from build123d import *

# Parameters (mm, degrees)
SKETCH_1_W          = 28
SKETCH_1_H          = 14
EXTRUDE_1_DEPTH     = 14
SKETCH_2_W          = 10
SKETCH_2_H          = 12
CUT_EXTRUDE_1_DEPTH = 25.3
SKETCH_3_R          = 2
CUT_EXTRUDE_2_DEPTH = 25.5
FILLET_4_R          = 2
SKETCH_4_W          = 9.3
SKETCH_4_H          = 14
EXTRUDE_2_DEPTH     = 5
SKETCH_5_W          = 5
SKETCH_5_H          = 14
EXTRUDE_3_DEPTH     = 5
SKETCH_6_R          = 1.48
CUT_EXTRUDE_3_DEPTH = 20


with BuildPart() as part:
    # 草图1 → 凸台-拉伸1 (new body)
    with BuildSketch(Plane(origin=(0, 0, 0), x_dir=(1, 0, 0), z_dir=(0, 1, 0))):
        Rectangle(SKETCH_1_W, SKETCH_1_H)
    extrude(amount=EXTRUDE_1_DEPTH)

    # 草图2 → 切除-拉伸1 (cut)
    with BuildSketch(Plane.ZY.offset(14)):
        with Locations((0, 7)):
            Rectangle(SKETCH_2_W, SKETCH_2_H)
    extrude(amount=-CUT_EXTRUDE_1_DEPTH, mode=Mode.SUBTRACT)

    # 草图3 → 切除-拉伸2 (cut)
    with BuildSketch(Plane(origin=(14, 0, 0), x_dir=(0, 0, -1), z_dir=(1, 0, 0))):
        with Locations((0, 10.5)):
            Circle(SKETCH_3_R)
        with Locations((0, 3.5)):
            Circle(SKETCH_3_R)
    extrude(amount=-CUT_EXTRUDE_2_DEPTH, mode=Mode.SUBTRACT)

    # 圆角4
    fillet_4_edges = [part.edges().sort_by_distance(p)[0] for p in [
        (14, 7, 7),
        (14, 7, -7),
    ]]
    fillet(fillet_4_edges, radius=FILLET_4_R)

    # 草图4 → 凸台-拉伸2 (add)
    with BuildSketch(Plane.XY.offset(7)):
        with Locations((2.35, 7)):
            Rectangle(SKETCH_4_W, SKETCH_4_H)
    extrude(amount=EXTRUDE_2_DEPTH)

    # 草图5 → 凸台-拉伸3 (add)
    with BuildSketch(Plane(origin=(0, 0, -7), x_dir=(-1, 0, 0), z_dir=(0, 0, -1))):
        with Locations((1.8, 7)):
            Rectangle(SKETCH_5_W, SKETCH_5_H)
    extrude(amount=EXTRUDE_3_DEPTH)

    # 草图6 → 切除-拉伸3 (cut)
    with BuildSketch(Plane(origin=(0, 14, 0), x_dir=(1, 0, 0), z_dir=(0, 1, 0))):
        with Locations(Location((2.7, -8.5, 0), (0, 0, 270))):
            Circle(SKETCH_6_R)
        with Locations(Location((-1.8, 8.5, 0), (0, 0, 270))):
            Circle(SKETCH_6_R)
    extrude(amount=-CUT_EXTRUDE_3_DEPTH, mode=Mode.SUBTRACT)


solid = part.part
Read the model definition and answer for the solid it produces. Units are mm, in the model's axes. A direction names the side the tool comes from. Give positions to 0.01 mm unless a question says otherwise; leave off trailing zeros. Write each loop counter-clockwise with the first axis right and the second up, starting at its lowest first coordinate (ties: lowest second). Pieces come first, ordered by that corner, then holes. Notation, with made-up numbers: (88.25, -7.5) - (105.25, -7.5) arc R23 cw to (105.25, 26.5) - close; hole circle Ø6 at (11, 81.25). An arc over 180 degrees is marked (long way). Use CSV: the item, a comma, the result in double quotes. Start each with the question number.
Item 1: The part is cut by section A-A, the plane x = -1.8. Give the vertices of the cut face in (y, z), and give its area (3 significant figures).
Item 2: The part is cut by section D-D, the plane z = 0. Give the vertices of the cut face in (x, y).
Item 3: Consider line 1 (Y direction, x = 13, z = 0); line 2 (Z direction, x = -8.75, y = 3.75); line 3 (Y direction, x = 4.75, z = -2.75). Determine where each line is inside the solid, lowest interval first.
Item 4: The part is cut by section C-C, the plane z = 8.5. Give the vertices of the cut face in (x, y), and give its area (3 significant figures).
Item 5: The mould has two halves that part along Y. Classify faces 6 (the flat face through (-2, 13, 0)), 7 (the flat face through (0, 0, 0)), 8 (the flat face through (-2, 7, -12)): pulls with the +Y half, pulls with the -Y half, needs draft (parallel to the pull), parting line crosses it, or undercut.
Item 6: Flat-ended cylindrical pins translate along their axes: P1, Ø2.5, axis at y = 9.5, z = 10, coming from the +X side; P2, Ø1.5, axis at y = 5.5, z = -10.5, coming from the +X side; P3, Ø3.5, axis at x = 5, y = 10, coming from the -Z side; P4, Ø3.5, axis at y = 10.5, z = 0, coming from the -X side. Find the tip coordinate at first contact, or state that the pin passes through.
Item 7: The part is cut by section B-B, the plane y = 3.5. Give the vertices of the cut face in (x, z).
Item 8: For faces 1 (the flat face through (-2, 7, 5)), 2 (the flat face through (0, 14, 0)), 3 (the flat face through (0.7, 7, -9)), 4 (the flat face through (-2.3, 7, 9)), 5 (the flat face through (7, 7, 9)), determine the directions among +Z, -Z, +X, -X, +Y, -Y from which every point of the face is accessible in a straight line to the end or side of a thin tool.
Taken from the geometry:
1,outline,"(0, -12) - (14, -12) - (14, -9.98) - (0, -9.98) - close; (0, -7.02) - (14, -7.02) - (14, 12) - (0, 12) - close; hole (1, -5) - (13, -5) - (13, 5) - (1, 5) - close"
1,area,"175 mm2"
2,outline,"(-14, 0) - (14, 0) - (14, 1.5) - (11.3, 1.5) - (11.3, 1) - (-14, 1) - close; (-14, 13) - (11.3, 13) - (11.3, 12.5) - (14, 12.5) - (14, 14) - (-14, 14) - close; (11.3, 5.5) - (14, 5.5) - (14, 8.5) - (11.3, 8.5) - close"
3,line 1,"0 to 1.5, 5.5 to 8.5, 12.5 to 14"
3,line 2,"-7 to -5, 5 to 7"
3,line 3,"0 to 1, 13 to 14"
4,outline,"(-2.3, 0) - (1.22, 0) - (1.22, 14) - (-2.3, 14) - close; (4.18, 0) - (7, 0) - (7, 14) - (4.18, 14) - close"
4,area,"88.8 mm2"
5,face 6,"undercut"
5,face 7,"pulls with the -Y half"
5,face 8,"needs draft"
6,P1,"x = 7"
6,P2,"x = 0.7"
6,P3,"z = -7"
6,P4,"through"
7,outline,"(-14, -7) - (-4.3, -7) - (-4.3, -12) - (0.7, -12) - (0.7, -7) - (12, -7) arc R2 ccw to (14, -5) - (14, -2) - (11.3, -2) - (11.3, -5) - (-14, -5) - close; (-14, 5) - (11.3, 5) - (11.3, 2) - (14, 2) - (14, 5) arc R2 ccw to (12, 7) - (7, 7) - (7, 12) - (-2.3, 12) - (-2.3, 7) - (-14, 7) - close; hole circle Ø2.96 at (-1.8, -8.5); hole circle Ø2.96 at (2.7, 8.5)"
8,face 1,"-X"
8,face 2,"+Z, -Z, +X, -X, +Y"
8,face 3,"-Z, +X, +Y, -Y"
8,face 4,"+Z, -X, +Y, -Y"
8,face 5,"+Z, +X, +Y, -Y"
